The listing builds one solid part. Answer for the finished solid, in the listing's coordinates (mm). A direction names the side the tool comes from. Coordinates: 2 decimals unless noted, no trailing zeros. Write each loop counter-clockwise with the first axis right and the second up, starting at its lowest first coordinate (ties: lowest second). Pieces come first, ordered by that corner, then holes.
from build123d import *

# Parameters (mm, degrees)
GRIPPING_RIBS_DEPTH = 2.1


with BuildPart() as part:
    # Sketch1 → Main Body (revolve)
    with BuildSketch(Plane.XY, mode=Mode.PRIVATE) as main_body_sk:
        Polygon((0, 3.1), (-3.9, 3.1), (-3.9, 0.2), (-3, 0.2), (-3, 0), (-2.5, 0), (-2.5, 2.1), (0, 2.1), align=None)
    revolve(main_body_sk.sketch.rotate(Axis((0, 0, 0), (0, 1, 0)), 270), axis=Axis((0, 0, 0), (0, 1, 0)))

    # Sketch2 → Gripping Ribs (add)
    with BuildSketch(Plane.XZ.offset(-2.1)):
        with BuildLine():
            Line((-0.7, 2.4), (0.7, 2.4))
            ThreePointArc((0.7, 2.4), (0, 2.5), (-0.7, 2.4))
        make_face()
        with BuildLine():
            ThreePointArc((-2.4, 0.7), (-2.5, 0), (-2.4, -0.7))
            Line((-2.4, -0.7), (-2.4, 0.7))
        make_face()
        with BuildLine():
            Line((2.4, 0.7), (2.4, -0.7))
            ThreePointArc((2.4, -0.7), (2.474873734, -0.353553391), (2.5, 0))
            ThreePointArc((2.5, 0), (2.474873734, 0.353553391), (2.4, 0.7))
        make_face()
        with BuildLine():
            ThreePointArc((-0.7, -2.4), (0, -2.5), (0.7, -2.4))
            Line((0.7, -2.4), (-0.7, -2.4))
        make_face()
    extrude(amount=GRIPPING_RIBS_DEPTH)


solid = part.part
Q1. The part is cut by section A-A, the plane y = 1.65. Write down the section's boundary in (x, z), then the cut area to 3 significant figures.
Answers below:
outline: circle Ø7.8 at (0, 0); hole (-2.4, -0.7) arc R2.5 ccw to (-0.7, -2.4) - (0.7, -2.4) arc R2.5 ccw to (2.4, -0.7) - (2.4, 0.7) arc R2.5 ccw to (0.7, 2.4) - (-0.7, 2.4) arc R2.5 ccw to (-2.4, 0.7) - close
area: 28.5 mm2
Q2. The part is cut by section C-C, the plane x = 0. Write down the section's boundary in (y, z), then the cut area to 3 significant figures.
Answers below:
outline: (0, -3) - (0.2, -3) - (0.2, -3.9) - (3.1, -3.9) - (3.1, 3.9) - (0.2, 3.9) - (0.2, 3) - (0, 3) - (0, 2.4) - (2.1, 2.4) - (2.1, -2.4) - (0, -2.4) - close
area: 13.7 mm2
Q3. Which of the six approach directions +Z, -Z, +X, -X, +Y, -Y give full straight-line access (tool end or side, diameter ignored) to faces 1 (the face through (0, 2.1, 0)), 2 (the face through (-2, 0, -2))?
Answers below:
face 1: -Y
face 2: +Z, -Z, +X, -X, -Y
Q4. The part is cut by section B-B, the plane z = 0. Write down the section's boundary in (x, y), then the cut area to 3 significant figures.
Answers below:
outline: (-3.9, 0.2) - (-3, 0.2) - (-3, 0) - (-2.4, 0) - (-2.4, 2.1) - (2.4, 2.1) - (2.4, 0) - (3, 0) - (3, 0.2) - (3.9, 0.2) - (3.9, 3.1) - (-3.9, 3.1) - close
area: 13.7 mm2
Q5. Determine the mould class of faces 3 (the face through (0, 3.1, 0)), 4 (the face through (0, 1, -2.4)), 5 (the face through (2.373, 1.63, 3.095)) for opening direction X: released by +X, released by -X, zero draft, split by the parting line, or undercut.
Answers below:
face 3: zero draft
face 4: undercut
face 5: split by the parting line
Q6. Given pin 1 (1 mm diameter, centred on x = 1, y = 2.5, fed in from -Z); pin 2 (1.1 mm diameter, centred on y = 1.5, z = -0.5, fed in from +X); pin 3 (0.7 mm diameter, centred on y = 1, z = -0.5, fed in from -X); pin 4 (1.4 mm diameter, centred on x = 1, z = 0, fed in from -Y), each flat-ended and moving along its own axis, determine where each tip first touches the part or whether it passes through.
Answers below:
pin 1: stops at z = -3.87
pin 2: stops at x = 3.9
pin 3: stops at x = -3.9
pin 4: stops at y = 2.1
Q7. Find the intervals of material crossed by probe 1 along Z at (x, y) = (2, 0.25); probe 2 along Y at (x, z) = (0.25, -1); probe 3 along Z at (x, y) = (0.25, 0.6), in increasing order.
Answers below:
probe 1: z = -3.35 to -1.5, 1.5 to 3.35
probe 2: y = 2.1 to 3.1
probe 3: z = -3.89 to -2.4, 2.4 to 3.89
Q8. The part is cut by section D-D, the plane x = 2.75. Write down the section's boundary in (y, z).
Answers below:
outline: (0, -1.2) - (0.2, -1.2) - (0.2, -2.77) - (3.1, -2.77) - (3.1, 2.77) - (0.2, 2.77) - (0.2, 1.2) - (0, 1.2) - close
